Work out the finished part from the listing and answer in its coordinate system (mm). A direction names the side the tool comes from. Give positions to 0.01 mm unless a question says otherwise; leave off trailing zeros. Loops run counter-clockwise (first coordinate to the right, second up) from the corner with the lowest first, then second, coordinate; pieces in that order, holes last. Notation, with made-up numbers: M 11,17.5 L 46,17.5 A23 cw 46,56.5 Z; hole C 62,53 d1. An arc over 180 degrees is marked long. Use a Markdown table: item, result.
```python
from build123d import *

# Parameters (mm, degrees)
SKETCH1_W             = 25.4
SKETCH1_H             = 25.4
BOSS_EXTRUDE1_DEPTH   = 6.35
CUT_EXTRUDE1_DEPTH    = 20.05
F_6_32_TAPPED_HOLE1_D = 2.7051
F_6_32_TAPPED_HOLE2_D = 2.7051


with BuildPart() as part:
    # Sketch1 → Boss-Extrude1 (new body)
    with BuildSketch(Plane.XY):
        Rectangle(SKETCH1_W, SKETCH1_H)
    extrude(amount=BOSS_EXTRUDE1_DEPTH)

    # Sketch2 → Cut-Extrude1 (cut, through all)
    with BuildSketch(Plane.XY.offset(6.35)):
        with BuildLine():
            Line((-1.5875, 9.323361062), (-1.5875, 1.740204949))
            Line((-1.5875, 1.740204949), (1.5875, 1.740204949))
            Line((1.5875, 1.740204949), (1.5875, 9.323361062))
            ThreePointArc((1.5875, 9.323361062), (0, 9.525), (-1.5875, 9.323361062))
        make_face()
        with BuildLine():
            Line((1.5875, 1.740204949), (-1.5875, 1.740204949))
            Line((-1.5875, 1.740204949), (-1.5875, 9.323361062))
            ThreePointArc((-1.5875, 9.323361062), (-3.888564967, -1.845115786), (6.35, 3.175))
            ThreePointArc((6.35, 3.175), (5.020115786, 7.063564967), (1.5875, 9.323361062))
            Line((1.5875, 9.323361062), (1.5875, 1.740204949))
        make_face()
        with BuildLine():
            Line((-1.5875, 12.7), (-1.5875, 9.323361062))
            ThreePointArc((-1.5875, 9.323361062), (0, 9.525), (1.5875, 9.323361062))
            Line((1.5875, 9.323361062), (1.5875, 12.7))
            Line((1.5875, 12.7), (-1.5875, 12.7))
        make_face()
    extrude(amount=-CUT_EXTRUDE1_DEPTH, mode=Mode.SUBTRACT)

    # #6-32 Tapped Hole1 (through all)
    with Locations(Plane(origin=(12.7, 0, 0), x_dir=(0, 0, -1), z_dir=(1, 0, 0))):
        with Locations((-3.175, 3.175)):
            Hole(F_6_32_TAPPED_HOLE1_D / 2)

    # #6-32 Tapped Hole2 (through all)
    with Locations(Plane.XY.offset(6.35)):
        with Locations((0, -9.525)):
            Hole(F_6_32_TAPPED_HOLE2_D / 2)


solid = part.part
```
(1) A cutting plane is placed at A-A (x = 0). Write down the section's boundary in (y, z) (3 decimals).
Entries:
| item | result |
|---|---|
| outline | M -12.7,0 L -10.878,0 L -10.878,6.35 L -12.7,6.35 Z; M -8.172,0 L -3.175,0 L -3.175,6.35 L -8.172,6.35 Z |
(2) Which of the six approach directions +Z, -Z, +X, -X, +Y, -Y give full straight-line access (tool end or side, diameter ignored) to faces 1 (the flat face through (-1.588, 11, 3)), 2 (the flat face through (7, 12.7, 3))?
Entries:
| item | result |
|---|---|
| face 1 | +Z, -Z, +Y |
| face 2 | +Z, -Z, +X, -X, +Y |
(3) A cutting plane is placed at B-B (y = 1). Write down the section's boundary in (x, z).
Entries:
| item | result |
|---|---|
| outline | M -12.7,0 L -5.97,0 L -5.97,6.35 L -12.7,6.35 Z; M 5.97,0 L 12.7,0 L 12.7,6.35 L 5.97,6.35 Z |
(4) Consider probe 1 along Z at (x, y) = (7.5, 3.25); probe 2 along Y at (x, z) = (0, 3) (3 decimals); probe 3 along X at (y, z) = (-9.5, 4.25). Determine where each line is inside the solid, lowest interval first. Write a range as [from, to].
Entries:
| item | result |
|---|---|
| probe 1 | z = [0, 1.82], [4.53, 6.35] |
| probe 2 | y = [-12.7, -10.878], [-8.172, -3.175] |
| probe 3 | x = [-12.7, -1.35], [1.35, 12.7] |
(5) Given P1, Ø14.5, axis at x = 0, y = 3.175, coming from the -Z side, flat-ended and moving along its own axis, determine where the tip first touches the part or whether it passes through.
Entries:
| item | result |
|---|---|
| P1 | stops at z = 0 |
(6) The mould has two halves that part along X. Classify faces 3 (the cylindrical face through (0.176, -8.184, 3.131)), 4 (the flat face through (0, -12.7, 3)), 5 (the flat face through (12.7, 0, 3)), 6 (the flat face through (1.588, 11, 3)): released by +X, released by -X, zero draft, split by the parting line, or undercut.
Entries:
| item | result |
|---|---|
| face 3 | undercut |
| face 4 | zero draft |
| face 5 | released by +X |
| face 6 | undercut |
